CAD build for the part. Positions are in the model's coordinates, mm. A direction names the side the tool comes from. Round coordinates to 2 decimals unless told otherwise and drop trailing zeros. Order: outer loops, then holes, each group sorted by start corner. A loop starts at its lowest first (then second) coordinate and runs counter-clockwise, first axis right, second up. Notation, with made-up numbers: (30.5, 51.5) - (62.5, 51.5) arc R10 ccw to (62.5, 63.5) - close; hole circle Ø3 at (81, -10). An arc over 180 degrees is marked (long way). Use one line per item in the form item = value. Start each with the question number.
from build123d import *

# Parameters (mm, degrees)
BOSS_EXTRUDE2_DEPTH = 100
BOSS_EXTRUDE3_DEPTH = 30
SKETCH10_R          = 7.5
CUT_EXTRUDE2_DEPTH  = 210
SKETCH15_R          = 1.5
CUT_EXTRUDE3_DEPTH  = 10
SKETCH16_W          = 20
SKETCH16_H          = 12
BOSS_EXTRUDE5_DEPTH = 2
SKETCH17_W          = 3
SKETCH17_H          = 12
BOSS_EXTRUDE6_DEPTH = 25
SKETCH19_R          = 3.5
CUT_EXTRUDE4_DEPTH  = 1
SKETCH20_R          = 1.55
CUT_EXTRUDE5_DEPTH  = 3
SKETCH21_W          = 45
SKETCH21_H          = 1.5
BOSS_EXTRUDE7_DEPTH = 35
SKETCH23_R          = 8.25
CUT_EXTRUDE6_DEPTH  = 40
CUT_EXTRUDE7_DEPTH  = 40
SKETCH26_W          = 50
SKETCH26_H          = 42
CUT_EXTRUDE8_DEPTH  = 5
FILLET1_R           = 7
FILLET3_R           = 7
FILLET4_R           = 7
SKETCH27_W          = 50.001655339
SKETCH27_H          = 42
CUT_EXTRUDE9_DEPTH  = 5
FILLET5_R           = 7
FILLET6_R           = 7
FILLET7_R           = 7


# Some blends are built 0.0001 mm under size
with BuildPart() as part:
    # Sketch3 → Boss-Extrude2 (new body)
    with BuildSketch(Plane.XY):
        Polygon((-106.54853621, -30.277349769), (-106.54853621, 11.722650231), (43.45146379, 11.722650231), (43.45146379, -30.277349769), (38.45146379, -30.277349769), (38.45146379, 4.722650231), (-101.54853621, 4.722650231), (-101.54853621, -30.277349769), align=None)
    extrude(amount=BOSS_EXTRUDE2_DEPTH)

    # Sketch4 → Boss-Extrude3 (add)
    with BuildSketch(Plane.XY.offset(100)):
        with BuildLine():
            Line((-102.69853621, -0.277349769), (-102.69853621, -20.277349769))
            ThreePointArc((-102.69853621, -20.277349769), (-104.04853621, -21.627349769), (-105.39853621, -20.277349769))
            Line((-105.39853621, -20.277349769), (-105.39853621, -0.277349769))
            ThreePointArc((-105.39853621, -0.277349769), (-104.04853621, 1.072650231), (-102.69853621, -0.277349769))
        make_face()
        with BuildLine():
            Line((-56.54853621, 9.572650231), (-6.54853621, 9.572650231))
            ThreePointArc((-6.54853621, 9.572650231), (-5.19853621, 8.222650231), (-6.54853621, 6.872650231))
            Line((-6.54853621, 6.872650231), (-56.54853621, 6.872650231))
            ThreePointArc((-56.54853621, 6.872650231), (-57.89853621, 8.222650231), (-56.54853621, 9.572650231))
        make_face()
        with BuildLine():
            Line((42.45146379, -0.277349769), (42.45146379, -20.277349769))
            ThreePointArc((42.45146379, -20.277349769), (40.95146379, -21.777349769), (39.45146379, -20.277349769))
            Line((39.45146379, -20.277349769), (39.45146379, -0.277349769))
            ThreePointArc((39.45146379, -0.277349769), (40.95146379, 1.222650231), (42.45146379, -0.277349769))
        make_face()
    extrude(amount=BOSS_EXTRUDE3_DEPTH)

    # Sketch10 → Cut-Extrude2 (cut)
    with BuildSketch(Plane(origin=(43.45146379, 0, 0), x_dir=(0, 0, -1), z_dir=(1, 0, 0))):
        with Locations((-45, -8.277349769)):
            Circle(SKETCH10_R)
    extrude(amount=-CUT_EXTRUDE2_DEPTH, mode=Mode.SUBTRACT)

    # Sketch15 → Cut-Extrude3 (cut)
    with BuildSketch(Plane(origin=(0, 11.722650231, 0), x_dir=(1, 0, 0), z_dir=(0, 1, 0))):
        with Locations(Location((-31.54853621, -4.714245873, 0), (0, 0, 270))):
            Circle(SKETCH15_R)
    extrude(amount=-CUT_EXTRUDE3_DEPTH, mode=Mode.SUBTRACT)

    # Sketch16 → Boss-Extrude5 (add)
    with BuildSketch(Plane.XZ.offset(-4.722650231)):
        with Locations((28.45146379, 69)):
            Rectangle(SKETCH16_W, SKETCH16_H)
    boss_extrude5 = extrude(amount=BOSS_EXTRUDE5_DEPTH)

    # Sketch17 → Boss-Extrude6 (add)
    with BuildSketch(Plane(origin=(0, 2.722650231, 0), x_dir=(-1, 0, 0), z_dir=(0, -1, 0))):
        with Locations((-19.95146379, -69)):
            Rectangle(SKETCH17_W, SKETCH17_H)
    boss_extrude6 = extrude(amount=BOSS_EXTRUDE6_DEPTH)

    # Sketch19 → Cut-Extrude4 (cut)
    with BuildSketch(Plane.ZY.offset(-18.45146379)):
        with Locations((69.485133357, 0.222650231)):
            Circle(SKETCH19_R)
        with Locations((69.485133357, -17.777349769)):
            Circle(SKETCH19_R)
    cut_extrude4 = extrude(amount=-CUT_EXTRUDE4_DEPTH, mode=Mode.SUBTRACT)

    # Sketch20 → Cut-Extrude5 (cut)
    with BuildSketch(Plane.ZY.offset(-19.45146379)):
        with Locations((69.485133357, 0.222650231)):
            Circle(SKETCH20_R)
        with Locations((69.485133357, -17.777349769)):
            Circle(SKETCH20_R)
    cut_extrude5 = extrude(amount=-CUT_EXTRUDE5_DEPTH, mode=Mode.SUBTRACT)

    # Mirror6: Boss-Extrude5, Boss-Extrude6, Cut-Extrude4, Cut-Extrude5 across plane
    add(boss_extrude5.mirror(Plane.ZY.offset(31.54853621)))
    add(boss_extrude6.mirror(Plane.ZY.offset(31.54853621)))
    add(cut_extrude4.mirror(Plane.ZY.offset(31.54853621)), mode=Mode.SUBTRACT)
    add(cut_extrude5.mirror(Plane.ZY.offset(31.54853621)), mode=Mode.SUBTRACT)

    # Sketch21 → Boss-Extrude7 (add)
    with BuildSketch(Plane.XZ.offset(-4.722650231)):
        with Locations((-31.54853621, 0.75)):
            Rectangle(SKETCH21_W, SKETCH21_H)
    extrude(amount=BOSS_EXTRUDE7_DEPTH)

    # Sketch23 → Cut-Extrude6 (cut)
    with BuildSketch(Plane(origin=(0, 0, 0), x_dir=(-1, 0, 0), z_dir=(0, 0, -1))):
        with Locations((44.54853621, -16.277349769)):
            Circle(SKETCH23_R)
        with Locations((18.54853621, -16.277349769)):
            Circle(SKETCH23_R)
    extrude(amount=-CUT_EXTRUDE6_DEPTH, mode=Mode.SUBTRACT)

    # Sketch24 → Cut-Extrude7 (cut)
    with BuildSketch(Plane(origin=(0, 0, 0), x_dir=(-1, 0, 0), z_dir=(0, 0, -1))):
        with BuildLine():
            Line((26.54853621, -23.095326639), (36.54853621, -23.095326639))
            ThreePointArc((36.54853621, -23.095326639), (39.773941895, -26.320732325), (36.54853621, -29.54613801))
            Line((36.54853621, -29.54613801), (26.54853621, -29.54613801))
            ThreePointArc((26.54853621, -29.54613801), (23.323130524, -26.320732325), (26.54853621, -23.095326639))
        make_face()
    extrude(amount=-CUT_EXTRUDE7_DEPTH, mode=Mode.SUBTRACT)

    # Sketch26 → Cut-Extrude8 (cut)
    with BuildSketch(Plane.ZY.offset(106.54853621)):
        with Locations((54.271655339, -9.277349769)):
            Rectangle(SKETCH26_W, SKETCH26_H)
    extrude(amount=-CUT_EXTRUDE8_DEPTH, mode=Mode.SUBTRACT)

    # Fillet1
    fillet1_edges = [part.edges().sort_by_distance(p)[0] for p in [
        (-101.54853621, 11.722650231, 54.271655339),
    ]]
    fillet(fillet1_edges, radius=FILLET1_R - 0.0001)  # a hair under: the kernel refuses the full size

    # Fillet3
    # the kernel refuses this fillet: 7 mm, written as the material it takes off along each edge
    with BuildSketch(Plane(origin=(-106.54853621, -47.777349769, 29.271655339), x_dir=(0, 0, -1), z_dir=(0, 1, 0))) as fillet3_piece_1_section:
        with BuildLine():
            CenterArc((FILLET3_R, -FILLET3_R), FILLET3_R, 90, 90)
            Line((0, -FILLET3_R), (0, 0))
            Line((0, 0), (FILLET3_R, 0))
        make_face()
    fillet3_piece_1 = extrude(amount=77, mode=Mode.PRIVATE)
    fillet3_piece_1 = fillet3_piece_1 - Plane(origin=(-94.54863621, 4.722750231, 27.624323614), x_dir=(0, 1, 0), z_dir=(0, 0, 1)) * Cylinder(6.9999, 182, mode=Mode.PRIVATE)
    add(fillet3_piece_1, mode=Mode.SUBTRACT)

    # Fillet4
    # the kernel refuses this fillet: 7 mm, written as the material it takes off along each edge
    with BuildSketch(Plane(origin=(-106.54853621, 29.222650231, 79.271655339), x_dir=(0, 0, 1), z_dir=(0, -1, 0))) as fillet4_piece_1_section:
        with BuildLine():
            CenterArc((FILLET4_R, -FILLET4_R), FILLET4_R, 90, 90)
            Line((0, -FILLET4_R), (0, 0))
            Line((0, 0), (FILLET4_R, 0))
        make_face()
    fillet4_piece_1 = extrude(amount=77, mode=Mode.PRIVATE)
    fillet4_piece_1 = fillet4_piece_1 - Plane(origin=(-94.54863621, 4.722750231, 80.918987064), x_dir=(0, 1, 0), z_dir=(0, 0, 1)) * Cylinder(6.9999, 182, mode=Mode.PRIVATE)
    add(fillet4_piece_1, mode=Mode.SUBTRACT)

    # Sketch27 → Cut-Extrude9 (cut)
    with BuildSketch(Plane(origin=(43.45146379, 0, 0), x_dir=(0, 0, -1), z_dir=(1, 0, 0))):
        with Locations((-54.27082767, -9.277349769)):
            Rectangle(SKETCH27_W, SKETCH27_H)
    extrude(amount=-CUT_EXTRUDE9_DEPTH, mode=Mode.SUBTRACT)

    # Fillet5
    fillet5_edges = [part.edges().sort_by_distance(p)[0] for p in [
        (38.45146379, 11.722650231, 54.270827669),
    ]]
    fillet(fillet5_edges, radius=FILLET5_R - 0.0001)  # a hair under: the kernel refuses the full size

    # Fillet6
    # the kernel refuses this fillet: 7 mm, written as the material it takes off along each edge
    with BuildSketch(Plane(origin=(43.45146379, -47.777349769, 29.27), x_dir=(0, 0, -1), z_dir=(0, 1, 0))) as fillet6_piece_1_section:
        with BuildLine():
            CenterArc((FILLET6_R, FILLET6_R), FILLET6_R, 180, 90)
            Line((0, FILLET6_R), (0, 0))
            Line((0, 0), (FILLET6_R, 0))
        make_face()
    fillet6_piece_1 = extrude(amount=77, mode=Mode.PRIVATE)
    fillet6_piece_1 = fillet6_piece_1 - Plane(origin=(31.45156379, 4.722750231, 27.622668275), x_dir=(0, 1, 0), z_dir=(0, 0, 1)) * Cylinder(6.9999, 182, mode=Mode.PRIVATE)
    add(fillet6_piece_1, mode=Mode.SUBTRACT)

    # Fillet7
    # the kernel refuses this fillet: 7 mm, written as the material it takes off along each edge
    with BuildSketch(Plane(origin=(43.45146379, 29.222650231, 79.271655339), x_dir=(-1, 0, 0), z_dir=(0, -1, 0))) as fillet7_piece_1_section:
        with BuildLine():
            CenterArc((FILLET7_R, -FILLET7_R), FILLET7_R, 90, 90)
            Line((0, -FILLET7_R), (0, 0))
            Line((0, 0), (FILLET7_R, 0))
        make_face()
    fillet7_piece_1 = extrude(amount=77, mode=Mode.PRIVATE)
    fillet7_piece_1 = fillet7_piece_1 - Plane(origin=(31.45156379, 4.722750231, 79.268302474), x_dir=(0, 1, 0), z_dir=(0, 0, 1)) * Cylinder(6.9999, 183, mode=Mode.PRIVATE)
    add(fillet7_piece_1, mode=Mode.SUBTRACT)


solid = part.part
(1) Slice it at A-A (z = 106.5). Give the cut face in (x, y).
(2) Flat gauge pins, fed straight in: P1, Ø10, axis at y = -7, z = 57, coming from the +X side; P2, Ø9.5, axis at x = 31, z = 68.5, coming from the -Y side; P3, Ø7.5, axis at y = 1, z = 69, coming from the -X side; P4, Ø3.5, axis at x = 20, z = 70.5, coming from the -Y side. Where does each tip first touch, or does it go through?
(3) Wall check: line 1 (X direction, y = -25.5, z = 13); line 2 (X direction, y = -20.5, z = 117); line 3 (Y direction, x = -55, z = 74). Give the ranges that are in metal, low to high. Write a range as [from, to].
(4) Mould opens along Y. For faces 4 (the cylindrical face through (18.944, -1.118, 72.718)), 5 (the cylindrical face through (-99.44, 9.73, 54.63)), 6 (the flat face through (-104, -30.277, 90)), 7 (the flat face through (-32, -9, 1.5)) say: pulls with the +Y half, pulls with the -Y half, needs draft (parallel to the pull), parting line crosses it, or undercut.
(5) Which spindle directions (+Z, -Z, +X, -X, +Y, -Y) get a long thin tool onto all of the face, cutting with end or side? Do faces 1 (the flat face through (19.451, -1, 71)), 2 (the flat face through (-81.549, -9, 69)), 3 (the flat face through (21, -5, 63)). Say none if no direction does.
(6) Slice it at C-C (x = -49). Give the cut face in (y, z).
(7) Slice it at B-B (x = 25.5). Give the cut face in (y, z).
Results list:
q1.outline = (-105.4, -20.28) arc R1.35 ccw to (-102.7, -20.28) - (-102.7, -0.28) arc R1.35 ccw to (-105.4, -0.28) - close; (-56.55, 6.87) - (-6.55, 6.87) arc R1.35 ccw to (-6.55, 9.57) - (-56.55, 9.57) arc R1.35 ccw to start; (39.45, -20.28) arc R1.5 ccw to (42.45, -20.28) - (42.45, -0.28) arc R1.5 ccw to (39.45, -0.28) - close
q2.P1 = through
q2.P2 = 2.72
q2.P3 = -101.55
q2.P4 = -22.28
q3.line_1 = [-106.55, -101.55], [38.45, 43.45]
q3.line_2 = [-105.38, -102.72], [39.47, 42.43]
q3.line_3 = [4.72, 11.72]
q4.face_4 = undercut
q4.face_5 = pulls with the +Y half
q4.face_6 = pulls with the -Y half
q4.face_7 = needs draft
q5.face_1 = none
q5.face_2 = +Z, -Z, -Y
q5.face_3 = -Z, +X, -X, -Y
q6.outline = (-30.28, 0) - (-23.22, 0) - (-23.22, 1.5) - (-30.28, 1.5) - close; (-9.33, 0) - (11.72, 0) - (11.72, 100) - (9.57, 100) - (9.57, 130) - (6.87, 130) - (6.87, 100) - (4.72, 100) - (4.72, 1.5) - (-9.33, 1.5) - close
q7.outline = (2.72, 63) - (4.72, 63) - (4.72, 0) - (11.72, 0) - (11.72, 100) - (4.72, 100) - (4.72, 75) - (2.72, 75) - close
